```python
from build123d import *

# Parameters (mm, degrees)
CROQUIS1_W                = 209.55
CROQUIS1_H                = 146.05
SALIENTE_EXTRUIR1_DEPTH   = 3.1242
CROQUIS2_R                = 1.3335
CORTAR_EXTRUIR1_DEPTH     = 128.750584639
CROQUIS9_R                = 1.27
CORTAR_EXTRUIR6_DEPTH     = 128.750584639
CORTAR_EXTRUIR2_DEPTH     = 128.750584639
CROQUIS5_R                = 1.651
DRIVER_DEPTH              = 128.750584639
CROQUIS6_R                = 1.651
RASPI_DEPTH               = 128.750584639
CROQUIS8_R                = 1.27
DIFERENCIAL_TRASERO_DEPTH = 128.750584639
CROQUIS7_R                = 1.5875
CROQUIS7_W                = 11.1125
CROQUIS7_H                = 2.9972
CORTAR_EXTRUIR7_DEPTH     = 128.750584639
CROQUIS10_R               = 1.651
CROQUIS10_W               = 22.606
CROQUIS10_H               = 11.9888
CORTAR_EXTRUIR10_DEPTH    = 128.750584639
CORTAR_EXTRUIR11_DEPTH    = 128.750584639
CROQUIS12_R               = 1.651
CORTAR_EXTRUIR12_DEPTH    = 128.750584639


with BuildPart() as part:
    # Croquis1 → Saliente-Extruir1 (new body)
    with BuildSketch(Plane.XY):
        Rectangle(CROQUIS1_W, CROQUIS1_H)
    extrude(amount=SALIENTE_EXTRUIR1_DEPTH)

    # Croquis2 → Cortar-Extruir1 (cut, through all)
    with BuildSketch(Plane.XY.offset(3.1242)):
        with BuildLine():
            ThreePointArc((80.5799125, 60.7314), (79.928852882, 61.877042778), (78.6114125, 61.904002767))
            Line((78.6114125, 61.904002767), (78.6114125, 59.558797233))
            ThreePointArc((78.6114125, 59.558797233), (79.928852882, 59.585757222), (80.5799125, 60.7314))
        make_face()
        with BuildLine():
            Line((78.6114125, 59.558797233), (78.6114125, 61.904002767))
            ThreePointArc((78.6114125, 61.904002767), (77.9129125, 60.7314), (78.6114125, 59.558797233))
        make_face()
        with Locations(Location((79.2464125, -60.7314, 0), (0, 0, 180))):
            Circle(CROQUIS2_R)
    extrude(amount=-CORTAR_EXTRUIR1_DEPTH, mode=Mode.SUBTRACT)

    # Croquis9 → Cortar-Extruir6 (cut, through all)
    with BuildSketch(Plane.XY.offset(3.1242)):
        with Locations((63.3206125, 37.6809)):
            Circle(CROQUIS9_R)
        with Locations((95.1722125, 37.6809)):
            Circle(CROQUIS9_R)
        with Locations(Location((95.1722125, -37.6809, 0), (0, 0, 180))):
            Circle(CROQUIS9_R)
        with Locations(Location((63.3206125, -37.6809, 0), (0, 0, 180))):
            Circle(CROQUIS9_R)
    extrude(amount=-CORTAR_EXTRUIR6_DEPTH, mode=Mode.SUBTRACT)

    # Croquis3 → Cortar-Extruir2 (cut, through all)
    with BuildSketch(Plane.XY.offset(3.1242)):
        with BuildLine():
            Line((38.1, 67.507041999), (38.1, 73.025))
            Line((38.1, 73.025), (31.75, 73.025))
            ThreePointArc((31.75, 73.025), (35.663372801, 71.675801268), (37.913779422, 68.201539629))
            ThreePointArc((37.913779422, 68.201539629), (38.003556568, 67.853397075), (38.1, 67.507041999))
        make_face()
        with BuildLine():
            Line((74.0870375, 73.025), (38.1, 73.025))
            Line((38.1, 73.025), (38.1, 67.507041999))
            ThreePointArc((38.1, 67.507041999), (44.836488972, 57.735545708), (56.09351875, 53.975))
            ThreePointArc((56.09351875, 53.975), (63.258442282, 54.43812298), (70.304123502, 55.81978439))
            ThreePointArc((70.304123502, 55.81978439), (73.03168636, 57.631625564), (74.0870375, 60.7314))
            Line((74.0870375, 60.7314), (74.0870375, 73.025))
        make_face()
        with BuildLine():
            Line((104.775, 73.025), (74.0870375, 73.025))
            Line((74.0870375, 73.025), (74.0870375, 60.7314))
            ThreePointArc((74.0870375, 60.7314), (77.605786537, 65.622974066), (83.362384549, 63.842336271))
            ThreePointArc((83.362384549, 63.842336271), (99.279214777, 33.668769191), (104.775, 5.82e-07))
            Line((104.775, 5.82e-07), (104.775, 73.025))
        make_face()
        with BuildLine():
            Line((104.775, -73.025), (104.775, 5.82e-07))
            ThreePointArc((104.775, 5.82e-07), (99.279214962, -33.668768639), (83.362384549, -63.842336271))
            ThreePointArc((83.362384549, -63.842336271), (77.605786537, -65.622974066), (74.0870375, -60.7314))
            Line((74.0870375, -60.7314), (74.0870375, -73.025))
            Line((74.0870375, -73.025), (104.775, -73.025))
        make_face()
        with BuildLine():
            Line((74.0870375, -73.025), (74.0870375, -60.7314))
            ThreePointArc((74.0870375, -60.7314), (73.03168636, -57.631625564), (70.304123502, -55.81978439))
            ThreePointArc((70.304123502, -55.81978439), (63.258442282, -54.43812298), (56.09351875, -53.975))
            ThreePointArc((56.09351875, -53.975), (44.836488972, -57.735545708), (38.1, -67.507041999))
            Line((38.1, -67.507041999), (38.1, -73.025))
            Line((38.1, -73.025), (74.0870375, -73.025))
        make_face()
        with BuildLine():
            ThreePointArc((37.913779422, -68.201539629), (35.663372801, -71.675801268), (31.75, -73.025))
            Line((31.75, -73.025), (38.1, -73.025))
            Line((38.1, -73.025), (38.1, -67.507041999))
            ThreePointArc((38.1, -67.507041999), (38.003556568, -67.853397075), (37.913779422, -68.201539629))
        make_face()
        with BuildLine():
            ThreePointArc((-104.775, 63.5), (-101.985192091, 70.235192091), (-95.25, 73.025))
            Line((-95.25, 73.025), (-104.775, 73.025))
            Line((-104.775, 73.025), (-104.775, 63.5))
        make_face()
        with BuildLine():
            Line((-104.775, -73.025), (-95.25, -73.025))
            ThreePointArc((-95.25, -73.025), (-101.985192091, -70.235192091), (-104.775, -63.5))
            Line((-104.775, -63.5), (-104.775, -73.025))
        make_face()
    extrude(amount=-CORTAR_EXTRUIR2_DEPTH, mode=Mode.SUBTRACT)

    # Croquis5 → Driver (cut, through all)
    with BuildSketch(Plane.XY.offset(3.1242)):
        with BuildLine():
            Line((12.47775, -19.2786), (-18.82775, -19.2786))
            ThreePointArc((-18.82775, -19.2786), (-19.389016008, -19.511083992), (-19.6215, -20.07235))
            Line((-19.6215, -20.07235), (-19.6215, -25.8826))
            ThreePointArc((-19.6215, -25.8826), (-20.55143597, -28.12766403), (-22.7965, -29.0576))
            Line((-22.7965, -29.0576), (-24.7015, -29.0576))
            ThreePointArc((-24.7015, -29.0576), (-28.293602448, -30.545497552), (-29.7815, -34.1376))
            Line((-29.7815, -34.1376), (-29.7815, -54.991))
            ThreePointArc((-29.7815, -54.991), (-28.293602448, -58.583102448), (-24.7015, -60.071))
            Line((-24.7015, -60.071), (-22.7965, -60.071))
            ThreePointArc((-22.7965, -60.071), (-20.55143597, -61.00093597), (-19.6215, -63.246))
            Line((-19.6215, -63.246), (-19.6215, -69.05625))
            ThreePointArc((-19.6215, -69.05625), (-19.389016008, -69.617516008), (-18.82775, -69.85))
            Line((-18.82775, -69.85), (12.47775, -69.85))
            ThreePointArc((12.47775, -69.85), (13.039016008, -69.617516008), (13.2715, -69.05625))
            Line((13.2715, -69.05625), (13.2715, -59.563))
            ThreePointArc((13.2715, -59.563), (14.350225725, -56.958725725), (16.9545, -55.88))
            Line((16.9545, -55.88), (19.05, -55.88))
            ThreePointArc((19.05, -55.88), (20.172532015, -55.415032015), (20.6375, -54.2925))
            Line((20.6375, -54.2925), (20.6375, -34.8361))
            ThreePointArc((20.6375, -34.8361), (20.172532015, -33.713567985), (19.05, -33.2486))
            Line((19.05, -33.2486), (16.9545, -33.2486))
            ThreePointArc((16.9545, -33.2486), (14.350225725, -32.169874275), (13.2715, -29.5656))
            Line((13.2715, -29.5656), (13.2715, -20.07235))
            ThreePointArc((13.2715, -20.07235), (13.039016008, -19.511083992), (12.47775, -19.2786))
        make_face()
        with Locations((17.0815, -24.7396)):
            Circle(CROQUIS5_R)
        with Locations((-23.0505, -24.6126)):
            Circle(CROQUIS5_R)
        with Locations(Location((17.0815, -64.389, 0), (0, 0, 180))):
            Circle(CROQUIS5_R)
        with Locations(Location((-23.0505, -64.516, 0), (0, 0, 180))):
            Circle(CROQUIS5_R)
    extrude(amount=-DRIVER_DEPTH, mode=Mode.SUBTRACT)

    # Croquis6 → RasPi (cut, through all)
    with BuildSketch(Plane.XY.offset(3.1242)):
        with Locations((-29.95, 48.8814)):
            Circle(CROQUIS6_R)
        with Locations((19.05, 48.8814)):
            Circle(CROQUIS6_R)
        with Locations((19.05, -9.1186)):
            Circle(CROQUIS6_R)
        with Locations((-29.95, -9.1186)):
            Circle(CROQUIS6_R)
    extrude(amount=-RASPI_DEPTH, mode=Mode.SUBTRACT)

    # Croquis8 → Diferencial trasero (cut, through all)
    with BuildSketch(Plane.XY.offset(3.1242)):
        with Locations((-93.98, 54.3306)):
            Circle(CROQUIS8_R)
        with Locations((-61.214, 28.0162)):
            Circle(CROQUIS8_R)
    extrude(amount=-DIFERENCIAL_TRASERO_DEPTH, mode=Mode.SUBTRACT)

    # Croquis7 → Cortar-Extruir7 (cut, through all)
    with BuildSketch(Plane.XY.offset(3.1242)):
        with Locations((-92.508859415, -52.4764)):
            Circle(CROQUIS7_R)
        with Locations((-71.871359415, -52.4764)):
            Circle(CROQUIS7_R)
        with Locations((-82.190109415, -52.4764)):
            Rectangle(CROQUIS7_W, CROQUIS7_H)
    extrude(amount=-CORTAR_EXTRUIR7_DEPTH, mode=Mode.SUBTRACT)

    # Croquis10 → Cortar-Extruir10 (cut, through all)
    with BuildSketch(Plane.XY.offset(3.1242)):
        with Locations((82.0674, 9.652)):
            Circle(CROQUIS10_R)
        with Locations((82.0674, 0)):
            Rectangle(CROQUIS10_W, CROQUIS10_H)
        with Locations((82.0674, -9.652)):
            Circle(CROQUIS10_R)
        Polygon((93.3704, -1.966579717), (93.3704, -2.54), (95.4024, -2.54), (95.4024, 2.54), (93.3704, 2.54), align=None)
    extrude(amount=-CORTAR_EXTRUIR10_DEPTH, mode=Mode.SUBTRACT)

    # Croquis11 → Cortar-Extruir11 (cut, through all)
    with BuildSketch(Plane.XY.offset(3.1242)):
        with BuildLine():
            Line((-61.62675, 63.8302), (-84.93125, 63.8302))
            ThreePointArc((-84.93125, 63.8302), (-85.492516008, 63.597716008), (-85.725, 63.03645))
            Line((-85.725, 63.03645), (-85.725, 52.0827))
            ThreePointArc((-85.725, 52.0827), (-85.957483992, 51.521433992), (-86.51875, 51.28895))
            Line((-86.51875, 51.28895), (-95.72625, 51.28895))
            ThreePointArc((-95.72625, 51.28895), (-96.287516008, 51.056466008), (-96.52, 50.4952))
            Line((-96.52, 50.4952), (-96.52, 30.7467))
            ThreePointArc((-96.52, 30.7467), (-96.287516008, 30.185433992), (-95.72625, 29.95295))
            Line((-95.72625, 29.95295), (-61.62675, 29.95295))
            ThreePointArc((-61.62675, 29.95295), (-61.065483992, 30.185433992), (-60.833, 30.7467))
            Line((-60.833, 30.7467), (-60.833, 63.03645))
            ThreePointArc((-60.833, 63.03645), (-61.065483992, 63.597716008), (-61.62675, 63.8302))
        make_face()
        with BuildLine():
            ThreePointArc((-95.25, 73.025), (-98.445006556, 72.473157644), (-101.2698, 70.881573881))
            ThreePointArc((-101.2698, 70.881573881), (-99.585538364, 71.085343471), (-98.679, 69.651311567))
            Line((-98.679, 69.651311567), (-98.679, 67.0052))
            ThreePointArc((-98.679, 67.0052), (-98.214032015, 65.882667985), (-97.0915, 65.4177))
            Line((-97.0915, 65.4177), (-49.4665, 65.4177))
            ThreePointArc((-49.4665, 65.4177), (-48.343967985, 65.882667985), (-47.879, 67.0052))
            Line((-47.879, 67.0052), (-47.879, 71.4375))
            ThreePointArc((-47.879, 71.4375), (-47.414032015, 72.560032015), (-46.2915, 73.025))
            Line((-46.2915, 73.025), (-95.25, 73.025))
        make_face()
        with BuildLine():
            ThreePointArc((-98.679, -69.651311567), (-99.585538364, -71.085343471), (-101.2698, -70.881573881))
            ThreePointArc((-101.2698, -70.881573881), (-98.445006556, -72.473157644), (-95.25, -73.025))
            Line((-95.25, -73.025), (-46.2915, -73.025))
            ThreePointArc((-46.2915, -73.025), (-47.414032015, -72.560032015), (-47.879, -71.4375))
            Line((-47.879, -71.4375), (-47.879, -67.0052))
            ThreePointArc((-47.879, -67.0052), (-48.343967985, -65.882667985), (-49.4665, -65.4177))
            Line((-49.4665, -65.4177), (-97.0915, -65.4177))
            ThreePointArc((-97.0915, -65.4177), (-98.214032015, -65.882667985), (-98.679, -67.0052))
            Line((-98.679, -67.0052), (-98.679, -69.651311567))
        make_face()
    extrude(amount=-CORTAR_EXTRUIR11_DEPTH, mode=Mode.SUBTRACT)

    # Croquis12 → Cortar-Extruir12 (cut, through all)
    with BuildSketch(Plane.XY.offset(3.1242)):
        with Locations((38.1, 38.1)):
            Circle(CROQUIS12_R)
        with Locations((-38.1, 38.1)):
            Circle(CROQUIS12_R)
        with Locations((-38.1, -38.1)):
            Circle(CROQUIS12_R)
        with Locations((38.1, -38.1)):
            Circle(CROQUIS12_R)
    extrude(amount=-CORTAR_EXTRUIR12_DEPTH, mode=Mode.SUBTRACT)


solid = part.part
```
The model under review builds one solid part; all positions refer to its coordinate system, in mm. A direction names the side the tool comes from. Round coordinates to 2 decimals unless told otherwise and drop trailing zeros.
1) Clearance check with flat-ended pins moving along their axes: P1, Ø0.9, axis at x = 81.5, z = 2, coming from the +Y side; P2, Ø1.5, axis at y = -52, z = 1, coming from the +X side (3 decimals). State where each tip first meets the part, or that it passes through.
Values follow:
P1: stops at y = 65.57
P2: stops at x = 91.545
2) The part is to be moulded in two halves that separate along X. For faces 3 (the face through (35.71, -71.64, 1.58)), 4 (the face through (77.521, 65.594, 1.584)), 5 (the face through (-1, 1, 3.124)), say which applies: pulls with the +X half, pulls with the -X half, needs draft (parallel to the pull), parting line crosses it, or undercut.
Values follow:
face 3: pulls with the +X half
face 4: undercut
face 5: needs draft
3) Tool access review of faces 1 (the face through (77.69, -65.65, 1.58)), 2 (the face through (-28.333, -58.543, 1.584)): name each direction out of +Z, -Z, +X, -X, +Y, -Y from which nothing blocks a thin tool from reaching the whole face with its end or side.
Values follow:
face 1: +Z, -Z, -Y
face 2: +Z, -Z
4) Consider section A-A on z = 1.1. Give the number of separate pieces and of enclosed holes in the cut face, then the cut area to 3 significant figures.
Values follow:
separate pieces: 1
enclosed holes: 28
area: 23,500 mm2
5) Wall thickness on line 1 along Y through (x, z) = (-84.5, 2.7) (3 decimals); line 2 along Y through (x, z) = (19.05, 2.05) (3 decimals); line 3 along Y through (x, z) = (-38.1, 2) (3 decimals): over which ranges is each line inside the solid? List them lowest first.
Values follow:
line 1: y = -65.418 to -53.975, -50.978 to 29.953, 63.83 to 65.418
line 2: y = -73.025 to -55.88, -33.249 to -10.77, -7.468 to 47.23, 50.532 to 73.025
line 3: y = -73.025 to -39.751, -36.449 to 36.449, 39.751 to 73.025
